Check sheet for the modelled part. Datum: model origin and axes. Units: mm. Coordinates: 2 decimals unless noted, no trailing zeros. Write each loop counter-clockwise with the first axis right and the second up, starting at its lowest first coordinate (ties: lowest second). Pieces come first, ordered by that corner, then holes. Notation, with made-up numbers: (15.5, 59) - (41.5, 59) arc R27 cw to (41.5, 85) - close; hole circle Ø2 at (27.25, 78). An arc over 180 degrees is marked (long way). Write each question's results on one line, items separated by ' | '.
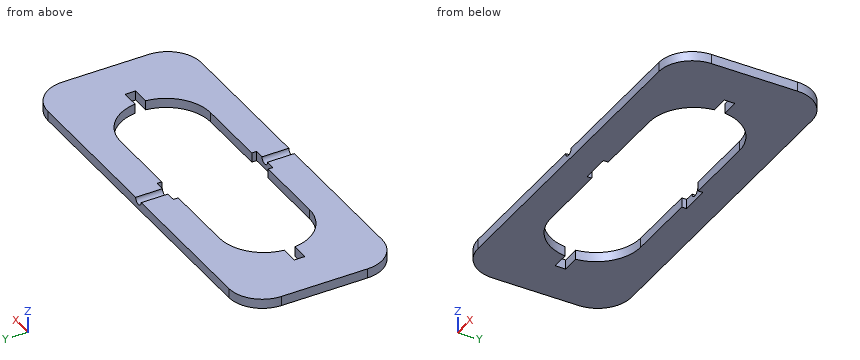
from build123d import *

# Parameters (mm, degrees)
BOSS_EXTRU_2_DEPTH      = 10
ENL_V_MAT_EXTRU_1_DEPTH = 10
ESQUISSE4_W             = 309
ESQUISSE4_H             = 11
ENL_V_MAT_EXTRU_2_DEPTH = 10
ESQUISSE5_W             = 30
ESQUISSE5_H             = 104
ENL_V_MAT_EXTRU_3_DEPTH = 10
ESQUISSE6_R             = 5
ENL_V_MAT_EXTRU_4_DEPTH = 161


with BuildPart() as part:
    # Esquisse2 → Boss.-Extru.2 (new body)
    with BuildSketch(Plane.XY):
        with BuildLine():
            Line((165, 80), (-165, 80))
            ThreePointArc((-165, 80), (-189.748737342, 69.748737342), (-200, 45))
            Line((-200, 45), (-200, -45))
            ThreePointArc((-200, -45), (-189.748737342, -69.748737342), (-165, -80))
            Line((-165, -80), (165, -80))
            ThreePointArc((165, -80), (189.748737342, -69.748737342), (200, -45))
            Line((200, -45), (200, 45))
            ThreePointArc((200, 45), (189.748737342, 69.748737342), (165, 80))
        make_face()
    extrude(amount=BOSS_EXTRU_2_DEPTH)

    # Esquisse3 → Enlèv. mat.-Extru.1 (cut)
    with BuildSketch(Plane.XY.offset(10)):
        with BuildLine():
            Line((90, 47), (-90, 47))
            ThreePointArc((-90, 47), (-122.880465325, 33.380465325), (-136.5, 0.5))
            Line((-136.5, 0.5), (-136.5, -0.5))
            ThreePointArc((-136.5, -0.5), (-122.880465325, -33.380465325), (-90, -47))
            Line((-90, -47), (90, -47))
            ThreePointArc((90, -47), (122.880465325, -33.380465325), (136.5, -0.5))
            Line((136.5, -0.5), (136.5, 0.5))
            ThreePointArc((136.5, 0.5), (122.880465325, 33.380465325), (90, 47))
        make_face()
    extrude(amount=-ENL_V_MAT_EXTRU_1_DEPTH, mode=Mode.SUBTRACT)

    # Esquisse4 → Enlèv. mat.-Extru.2 (cut)
    with BuildSketch(Plane.XY.offset(10)):
        Rectangle(ESQUISSE4_W, ESQUISSE4_H)
    extrude(amount=-ENL_V_MAT_EXTRU_2_DEPTH, mode=Mode.SUBTRACT)

    # Esquisse5 → Enlèv. mat.-Extru.3 (cut)
    with BuildSketch(Plane.XY.offset(10)):
        Rectangle(ESQUISSE5_W, ESQUISSE5_H)
    extrude(amount=-ENL_V_MAT_EXTRU_3_DEPTH, mode=Mode.SUBTRACT)

    # Esquisse6 → Enlèv. mat.-Extru.4 (cut, through all)
    with BuildSketch(Plane.XZ.offset(80)):
        with Locations((0, 10)):
            Circle(ESQUISSE6_R)
    extrude(amount=-ENL_V_MAT_EXTRU_4_DEPTH, mode=Mode.SUBTRACT)


solid = part.part
1. Sectioned sample at B-B (y = 13.5). Record the cut outline in (x, z).
Values follow:
outline: (-200, 0) - (-134.65, 0) - (-134.65, 10) - (-200, 10) - close; (134.65, 0) - (200, 0) - (200, 10) - (134.65, 10) - close
2. Sectioned sample at C-C (y = -57). Record the cut outline in (x, z), then the cut area to 3 significant figures.
Values follow:
outline: (-197.88, 0) - (197.88, 0) - (197.88, 10) - (5, 10) arc R5 cw to (-5, 10) - (-197.88, 10) - close | area: 3,920 mm^2
3. Material ranges on L1, parallel to Y at x = 40, z = 1.5; L2, parallel to Y at x = -140, z = 8.5; L3, parallel to X at y = 8, z = 0.5, recorded low to high. Write a range as [from, to].
Values follow:
L1: y = [-80, -47], [47, 80] | L2: y = [-80, -5.5], [5.5, 80] | L3: x = [-200, -135.89], [135.89, 200]
4. Go/stop test with flat-tipped pins: pin 1 (1.5 mm diameter, centred on y = -50, z = 3, fed in from +X); pin 2 (2.5 mm diameter, centred on y = -49.5, z = 5, fed in from +X); pin 3 (2.5 mm diameter, centred on y = 49, z = 5, fed in from -X). Record where each tip stops, or that it passes through.
Values follow:
pin 1: stops at x = 199.74 | pin 2: stops at x = 199.85 | pin 3: stops at x = -199.89
5. Sectioned sample at D-D (y = 60.5). Record the cut outline in (x, z), then the cut area to 3 significant figures.
Values follow:
outline: (-196.38, 0) - (196.38, 0) - (196.38, 10) - (5, 10) arc R5 cw to (-5, 10) - (-196.38, 10) - close | area: 3,890 mm^2
6. Sectioned sample at A-A (x = -36). Record the cut outline in (y, z), then the cut area to 3 significant figures.
Values follow:
outline: (-80, 0) - (-47, 0) - (-47, 10) - (-80, 10) - close; (47, 0) - (80, 0) - (80, 10) - (47, 10) - close | area: 660 mm^2
